from build123d import *

# Parameters (mm, degrees)
F0_W     = 40
F0_H     = 45
F1_DEPTH = 10
F2_R     = 1.5
F3_DEPTH = 25
F4_R     = 2
F5_DEPTH = 25


with BuildPart() as f1:
    # F0 (on Top) → F1 (new body)
    with BuildSketch(Plane.XY):
        Rectangle(F0_W, F0_H)
    extrude(amount=F1_DEPTH)

    # F2 (on face) → F3 (cut)
    with BuildSketch(Plane.XY.offset(10)):
        with Locations((0, 16.5)):
            Circle(F2_R)
    extrude(amount=-F3_DEPTH, mode=Mode.SUBTRACT)

    # F4 (on face) → F5 (cut)
    with BuildSketch(Plane.XY.offset(10)):
        with Locations((16, -12.5)):
            Circle(F4_R)
        with Locations((-16, -12.5)):
            Circle(F4_R)
    extrude(amount=-F5_DEPTH, mode=Mode.SUBTRACT)


solid = f1.part
The listing builds one solid part. Answer for the finished solid, in the listing's coordinates (mm). Round coordinates to 2 decimals unless told otherwise and drop trailing zeros. Write each loop counter-clockwise with the first axis right and the second up, starting at its lowest first coordinate (ties: lowest second). Pieces come first, ordered by that corner, then holes. Notation, with made-up numbers: (76.25, -17.75) - (104.25, -17.75) arc R29 cw to (104.25, 11.25) - close; hole circle Ø7 at (-5.75, 70). An arc over 180 degrees is marked (long way). Use a Markdown table: item, result. Add a question column.
1. For a pull along X with two mould halves and no side action, classify faces 1 (the face through (20, 0, 5)), 2 (the face through (0, 0, 10)), 3 (the face through (14.526, -11.148, 5.07)) as +X half, -X half, draft (parallel to the pull), parting line (faces both ways), or undercut.
2. The part is cut by section A-A (y = -12.5). Write down the section's boundary in (x, z).
3. Consider line 1 (Y direction, x = 0, z = 2.5); line 2 (Y direction, x = 16, z = 7); line 3 (X direction, y = -11, z = 6). Determine where each line is inside the solid, lowest interval first.
4. The part is cut by section B-B (x = 0). Write down the section's boundary in (y, z), and give its area (3 significant figures).
5. The part is cut by section C-C (x = 16). Write down the section's boundary in (y, z).
6. A flat-ended cylindrical pin translates along its axis: P1, Ø3.5, axis at x = -16, y = -12.5, coming from the +Z side. Find the tip coordinate at first contact, or state that the pin passes through.
Reported:
| question | item | result |
|---|---|---|
| 1 | face 1 | +X half |
| 1 | face 2 | draft |
| 1 | face 3 | undercut |
| 2 | outline | (-20, 0) - (-18, 0) - (-18, 10) - (-20, 10) - close; (-14, 0) - (14, 0) - (14, 10) - (-14, 10) - close; (18, 0) - (20, 0) - (20, 10) - (18, 10) - close |
| 3 | line 1 | -22.5 to 15, 18 to 22.5 |
| 3 | line 2 | -22.5 to -14.5, -10.5 to 22.5 |
| 3 | line 3 | -20 to -17.32, -14.68 to 14.68, 17.32 to 20 |
| 4 | outline | (-22.5, 0) - (15, 0) - (15, 10) - (-22.5, 10) - close; (18, 0) - (22.5, 0) - (22.5, 10) - (18, 10) - close |
| 4 | area | 420 mm^2 |
| 5 | outline | (-22.5, 0) - (-14.5, 0) - (-14.5, 10) - (-22.5, 10) - close; (-10.5, 0) - (22.5, 0) - (22.5, 10) - (-10.5, 10) - close |
| 6 | P1 | through |
